Could you check a few things on this model? Use its own coordinates, in mm. Face numbers are marked on the shaded views. Coordinates: 2 decimals unless noted, no trailing zeros. Write each loop counter-clockwise with the first axis right and the second up, starting at its lowest first coordinate (ties: lowest second). Pieces come first, ordered by that corner, then holes. Notation, with made-up numbers: (23, 57) - (69, 57) arc R15 cw to (69, 64) - close; hole circle Ø10 at (9, 84). An arc over 180 degrees is marked (long way). Answer as a JSON object with one key per item and string values. Group by question number.
1) We'd pull the mould along Z, two halves only. Please class the marked faces 1 and 2: released by +Z, released by -Z, zero draft, split by the parting line, or undercut.
2) If we section it at B-B (x = -36.5): Write out the boundary of the cut face in (y, z).
3) Please list where these lines run through material, in increasing order: line 1 along Z through (x, y) = (-44, -8.5); line 2 along Y through (x, z) = (-51, -20); line 3 along X through (y, z) = (-9.5, 13).
4) If we section it at A-A (z = 49): Write out the boundary of the cut face in (x, y).
5) Will this pin go through, and if not, where does the flat tip stop? pin 1 Ø5 at (x, z) = (27, 48) entering from -Y.
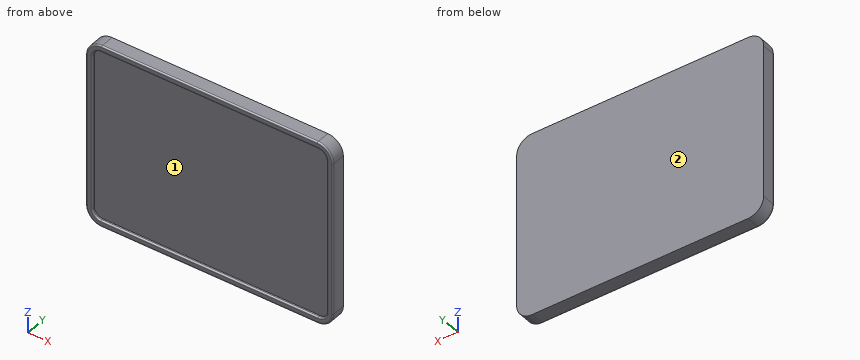
```python
from build123d import *

# Parameters (mm, degrees)
F1_DEPTH = 10
F3_DEPTH = 2
F4_R     = 1


with BuildPart() as f1:
    # F0 (on Front) → F1 (new body)
    with BuildSketch(Plane.XZ):
        with BuildLine():
            ThreePointArc((87, 54), (83.778175, 61.778175), (76, 65))
            Line((76, 65), (-76, 65))
            ThreePointArc((-76, 65), (-83.778175, 61.778175), (-87, 54))
            Line((-87, 54), (-87, -54))
            ThreePointArc((-87, -54), (-83.778175, -61.778175), (-76, -65))
            Line((-76, -65), (76, -65))
            ThreePointArc((76, -65), (83.778175, -61.778175), (87, -54))
            Line((87, -54), (87, 54))
        make_face()
        with BuildLine():
            Line((-76.5, 60.5), (76.5, 60.5))
            ThreePointArc((76.5, 60.5), (80.742641, 58.742641), (82.5, 54.5))
            Line((82.5, 54.5), (82.5, -54.5))
            ThreePointArc((82.5, -54.5), (80.742641, -58.742641), (76.5, -60.5))
            Line((76.5, -60.5), (-76.5, -60.5))
            ThreePointArc((-76.5, -60.5), (-80.742641, -58.742641), (-82.5, -54.5))
            Line((-82.5, -54.5), (-82.5, 54.5))
            ThreePointArc((-82.5, 54.5), (-80.742641, 58.742641), (-76.5, 60.5))
        make_face(mode=Mode.SUBTRACT)
        with BuildLine():
            ThreePointArc((82.5, 54.5), (80.742641, 58.742641), (76.5, 60.5))
            Line((76.5, 60.5), (-76.5, 60.5))
            ThreePointArc((-76.5, 60.5), (-80.742641, 58.742641), (-82.5, 54.5))
            Line((-82.5, 54.5), (-82.5, -54.5))
            ThreePointArc((-82.5, -54.5), (-80.742641, -58.742641), (-76.5, -60.5))
            Line((-76.5, -60.5), (76.5, -60.5))
            ThreePointArc((76.5, -60.5), (80.742641, -58.742641), (82.5, -54.5))
            Line((82.5, -54.5), (82.5, 54.5))
        make_face()
    extrude(amount=F1_DEPTH)

    # F2 (on face) → F3 (cut)
    with BuildSketch(Plane.XZ.offset(10)):
        with BuildLine():
            Line((76.5, 60.5), (-76.5, 60.5))
            ThreePointArc((-76.5, 60.5), (-80.742641, 58.742641), (-82.5, 54.5))
            Line((-82.5, 54.5), (-82.5, -54.5))
            ThreePointArc((-82.5, -54.5), (-80.742641, -58.742641), (-76.5, -60.5))
            Line((-76.5, -60.5), (76.5, -60.5))
            ThreePointArc((76.5, -60.5), (80.742641, -58.742641), (82.5, -54.5))
            Line((82.5, -54.5), (82.5, 54.5))
            ThreePointArc((82.5, 54.5), (80.742641, 58.742641), (76.5, 60.5))
        make_face()
    extrude(amount=-F3_DEPTH, mode=Mode.SUBTRACT)

    # F4
    f4_edges = [f1.edges().sort_by_distance(p)[0] for p in [
        (83.778175, -10, 61.778175),
        (87, -10, 0),
        (0, -10, 65),
        (83.778175, -10, -61.778175),
        (-83.778175, -10, 61.778175),
        (0, -10, -65),
        (-87, -10, 0),
        (-83.778175, -10, -61.778175),
        (0, -10, 60.5),
        (-80.742641, -10, 58.742641),
        (-82.5, -10, 0),
        (-80.742641, -10, -58.742641),
        (0, -10, -60.5),
        (80.742641, -10, -58.742641),
        (82.5, -10, 0),
        (80.742641, -10, 58.742641),
    ]]
    fillet(f4_edges, radius=F4_R)


solid = f1.part
```
Here are the results:
{
 "1": {"face 1": "undercut", "face 2": "zero draft"},
 "2": {"outline": "(-10, -64) arc R1 ccw to (-9, -65) - (0, -65) - (0, 65) - (-9, 65) arc R1 ccw to (-10, 64) - (-10, 61.5) arc R1 ccw to (-9, 60.5) - (-8, 60.5) - (-8, -60.5) - (-9, -60.5) arc R1 ccw to (-10, -61.5) - close"},
 "3": {"line 1": "z = -65 to -60.5, 60.5 to 65", "line 2": "y = -8 to 0", "line 3": "x = -86.87 to -82.63, 82.63 to 86.87"},
 "4": {"outline": "(-87, -9) arc R1 ccw to (-86, -10) - (-83.5, -10) arc R1 ccw to (-82.5, -9) - (-82.5, -8) - (82.5, -8) - (82.5, -9) arc R1 ccw to (83.5, -10) - (86, -10) arc R1 ccw to (87, -9) - (87, 0) - (-87, 0) - close"},
 "5": {"pin 1": "stops at y = -8"}
}
